Source: CAD feature listing. Evaluate the final solid. Frame: model axes, mm. A direction names the side the tool comes from. Give positions to 0.01 mm unless a question says otherwise; leave off trailing zeros. Order: outer loops, then holes, each group sorted by start corner. A loop starts at its lowest first (then second) coordinate and runs counter-clockwise, first axis right, second up.
from build123d import *

# Parameters (mm, degrees)
SKETCH1_R            = 40
SKETCH1_R_2          = 25
BOSS_EXTRUDE1_DEPTH  = 35
SKETCH2_R            = 40
BOSS_EXTRUDE2_DEPTH  = 5
BOSS_EXTRUDE3_START  = 5
SKETCH4_R            = 40
SKETCH4_R_2          = 30
BOSS_EXTRUDE3_DEPTH  = 5
SKETCH6_R            = 5
SKETCH6_R_2          = 3
HUB_DEPTH            = 30
FILLET1_DESIGN_R     = 5
HUB_HOLES_DEPTH      = 10
HUB_HOLES_DEPTH_BACK = 10
SKETCH8_R            = 1.5


with BuildPart() as part:
    # Sketch1 → Boss-Extrude1 (new body)
    with BuildSketch(Plane.XY):
        Circle(SKETCH1_R)
        Circle(SKETCH1_R_2, mode=Mode.SUBTRACT)
    extrude(amount=BOSS_EXTRUDE1_DEPTH)

    # Sketch2 → Boss-Extrude2 (add)
    with BuildSketch(Plane(origin=(0, 0, 0), x_dir=(-1, 0, 0), z_dir=(0, 0, -1))):
        with Locations(Location((0, 0, 0), (0, 0, 180))):
            Circle(SKETCH2_R)
    extrude(amount=-BOSS_EXTRUDE2_DEPTH)

    # Sketch4 → Boss-Extrude3 (add)
    with BuildSketch(Plane(origin=(0, 0, 0), x_dir=(-1, 0, 0), z_dir=(0, 0, -1)).offset(BOSS_EXTRUDE3_START)):
        Circle(SKETCH4_R)
        Circle(SKETCH4_R_2, mode=Mode.SUBTRACT)
    extrude(amount=-BOSS_EXTRUDE3_DEPTH)

    # Sketch6 → hub (add)
    with BuildSketch(Plane.XY.offset(5)):
        with Locations(Location((0, 0, 0), (0, 0, 180))):
            Circle(SKETCH6_R)
        Circle(SKETCH6_R_2, mode=Mode.SUBTRACT)
    extrude(amount=HUB_DEPTH)

    # Fillet1 design
    fillet1_design_edges = [part.edges().sort_by_distance(p)[0] for p in [
        (40, 0, -5),
        (30, 0, -5),
        (-40, 0, 35),
        (-25, 0, 35),
    ]]
    fillet(fillet1_design_edges, radius=FILLET1_DESIGN_R - 0.0001)  # a hair under: the kernel refuses the full size

    # Sketch8 → hub holes (cut, two sides: drawn at the far end of the back side and taken through both)
    with BuildSketch(Plane(origin=(0, 0, 0), x_dir=(1, 0, 0), z_dir=(0, 1, 0)).offset(-HUB_HOLES_DEPTH_BACK)):
        with Locations(Location((0, -30.243060778, 0), (0, 0, 90))):
            Circle(SKETCH8_R)
    extrude(amount=HUB_HOLES_DEPTH + HUB_HOLES_DEPTH_BACK, mode=Mode.SUBTRACT)


solid = part.part
(1) Pin query (flat end, axial travel): pin 1 Ø10 at (y, z) = (-3, 18) entering from +X; pin 2 Ø1.5 at (x, y) = (20, 16) entering from -Z; pin 3 Ø3 at (y, z) = (27, 22.5) entering from +X; pin 4 Ø10 at (y, z) = (-24.5, 20) entering from +X. Return the tip coordinate at first contact, or that it passes through.
(2) Access query for faces 1 (the flat face through (-0.3, 5.2, 5)), 2 (the flat face through (0, 0, 0)), 3 (the cylindrical face through (-0.07, -3.82, 31.74)). Directions: +Z, -Z, +X, -X, +Y, -Y. A direction counts if a zero-diameter tool reaches every point of the face in a straight line with its end or side. Return the directions, or none.
(3) Draft query along X for faces 4 (the flat face through (0, 0, 5)), 5 (the flat face through (26, 16, 35)), 6 (the cylindrical face through (-4.77, -1.5, 19.79)). Return one class per face: +X half, -X half, draft (parallel to the pull), parting line (faces both ways), or undercut.
(4) Section B-B, the plane x = 0. Count the separate pieces of the cut face and the enclosed holes in it, plus the area to 3 significant figures.
(5) Section A-A, the plane z = 18. Return loops of the section in (x, y), plus the area to 3 significant figures.
(6) Line query: line 1 along Y through (x, z) = (0, 19.75); line 2 along Y through (x, z) = (4.5, 22.5); line 3 along Z through (x, y) = (-20, -1.5). Output: solid intervals per line, ascending.
Checks:
1. pin 1: stops at x = 40
1. pin 2: stops at z = 0
1. pin 3: stops at x = 30.82
1. pin 4: stops at x = 34.92
2. face 1: +Z
2. face 2: -Z
2. face 3: none
3. face 4: undercut
3. face 5: draft
3. face 6: undercut
4. separate pieces: 3
4. enclosed holes: 0
4. area: 1,470 mm2
5. outline: circle Ø80 at (0, 0); circle Ø10 at (0, 0); hole circle Ø50 at (0, 0); hole circle Ø6 at (0, 0)
5. area: 3,110 mm2
6. line 1: y = -40 to -25, -5 to -3, 3 to 5, 25 to 40
6. line 2: y = -39.75 to -24.59, -2.18 to 2.18, 24.59 to 39.75
6. line 3: z = 0 to 5
